Read the model definition and answer for the solid it produces. Units are mm, in the model's axes. A direction names the side the tool comes from. Round coordinates to 2 decimals unless told otherwise and drop trailing zeros. Order: outer loops, then holes, each group sorted by start corner. A loop starts at its lowest first (then second) coordinate and runs counter-clockwise, first axis right, second up. Notation, with made-up numbers: (19.25, 78.25) -> (41.25, 78.25) arc R27 ccw to (41.25, 113.25) -> close; hole circle Ø10 at (62.25, 25). An arc over 180 degrees is marked (long way). Answer as a JSON object with one key per item and string values. Group by question number.
Item 1: Consider probe 1 along Y at (x, z) = (-3.5, -12); probe 2 along Y at (x, z) = (7.5, 8.5); probe 3 along Z at (x, y) = (-3.25, 1.2). Determine where each line is inside the solid, lowest interval first. Write a range as from..to.
Item 2: Section C-C, the plane x = 4 is taken. Write down the section's boundary in (y, z).
Item 3: The mould has two halves that part along Z. Classify faces 1 (the cylindrical face through (0.1, 1.4, -14.5)), 2 (the flat face through (12.5, 1, 0)), 3 (the cylindrical face through (0.11, 0.74, -11.01)): pulls with the +Z half, pulls with the -Z half, needs draft (parallel to the pull), parting line crosses it, or undercut.
Item 4: Section D-D, the plane z = -3.75 is taken. Write down the section's boundary in (x, y).
Item 5: For faces 4 (the flat face through (0, 0, 0)), 5 (the flat face through (8, 0, -13)), 6 (the flat face through (-8, 0, -13)), 7 (the cylindrical face through (11.297, 1.521, 8.859)), 8 (the flat face through (0, 3, 0)), determine the directions among +Z, -Z, +X, -X, +Y, -Y from which every point of the face is accessible in a straight line to the end or side of a thin tool.
Item 6: Section B-B, the plane y = 1.5 is taken. Write down the section's boundary in (x, z).
Item 7: Section A-A, the plane z = -12 is taken. Write down the section's boundary in (x, y).
Item 8: Given P1, Ø6, axis at x = 6, z = 1.5, coming from the -Y side; P2, Ø1.3, axis at y = 2, z = -11.5, coming from the +X side; P3, Ø3, axis at y = 1.5, z = -12, coming from the -X side; P4, Ø1, axis at x = 5.5, z = -11.5, coming from the +Y side, each flat-ended and moving along its own axis, determine where each tip first touches the part or whether it passes through.
from build123d import *

# Parameters (mm, degrees)
SKETCH2_W           = 25
SKETCH2_H           = 20
BOSS_EXTRUDE1_DEPTH = 3
FILLET1_R           = 4
SKETCH4_R           = 2.5
BOSS_EXTRUDE2_DEPTH = 8
SKETCH5_R           = 1.25
CUT_EXTRUDE1_DEPTH  = 16


with BuildPart() as part:
    # Sketch2 → Boss-Extrude1 (new body)
    with BuildSketch(Plane(origin=(0, 0, 0), x_dir=(1, 0, 0), z_dir=(0, 1, 0))):
        Rectangle(SKETCH2_W, SKETCH2_H)
    extrude(amount=BOSS_EXTRUDE1_DEPTH)

    # Fillet1
    fillet1_edges = [part.edges().sort_by_distance(p)[0] for p in [
        (12.5, 1.5, 10),
        (-12.5, 1.5, 10),
        (-12.5, 1.5, -10),
        (12.5, 1.5, -10),
    ]]
    fillet(fillet1_edges, radius=FILLET1_R)

    # Sketch4 → Boss-Extrude2 (add, symmetric)
    with BuildSketch(Plane(origin=(0, 0, 0), x_dir=(0, 0, -1), z_dir=(1, 0, 0))):
        with Locations((12, 1.5)):
            Circle(SKETCH4_R)
    extrude(amount=BOSS_EXTRUDE2_DEPTH, both=True)

    # Sketch5 → Cut-Extrude1 (cut)
    with BuildSketch(Plane(origin=(8, 0, 0), x_dir=(0, 0, -1), z_dir=(1, 0, 0))):
        with Locations((12, 1.5)):
            Circle(SKETCH5_R)
    extrude(amount=-CUT_EXTRUDE1_DEPTH, mode=Mode.SUBTRACT)


solid = part.part
Values found:
{
 "1": {"probe 1": "-1..0.25, 2.75..4", "probe 2": "0..3", "probe 3": "-14.48..-13.21, -10.79..10"},
 "2": {"outline": "(0, -10) arc R2.5 ccw (long way) to (3, -10) -> (3, 10) -> (0, 10) -> close; hole circle Ø2.5 at (1.5, -12)"},
 "3": {"face 1": "parting line crosses it", "face 2": "needs draft", "face 3": "undercut"},
 "4": {"outline": "(-12.5, 0) -> (12.5, 0) -> (12.5, 3) -> (-12.5, 3) -> close"},
 "5": {"face 4": "+Z, +X, -X, -Y", "face 5": "-Z, +X, +Y, -Y", "face 6": "-Z, -X, +Y, -Y", "face 7": "+Z, +X, +Y, -Y", "face 8": "+Z, +X, -X, +Y"},
 "6": {"outline": "(-12.5, -6) arc R4 ccw to (-8.5, -10) -> (-8, -10) -> (-8, -10.75) -> (8, -10.75) -> (8, -10) -> (8.5, -10) arc R4 ccw to (12.5, -6) -> (12.5, 6) arc R4 ccw to (8.5, 10) -> (-8.5, 10) arc R4 ccw to (-12.5, 6) -> close; (-8, -14.5) -> (8, -14.5) -> (8, -13.25) -> (-8, -13.25) -> close"},
 "7": {"outline": "(-8, -1) -> (8, -1) -> (8, 0.25) -> (-8, 0.25) -> close; (-8, 2.75) -> (8, 2.75) -> (8, 4) -> (-8, 4) -> close"},
 "8": {"P1": "y = 0", "P2": "x = 8", "P3": "x = -8", "P4": "y = 4"}
}
